Study the drawing (mm; zero at the part's minimum x, y, z) and answer. A direction names the side the tool comes from. Coordinates: 2 decimals unless noted, no trailing zeros. Write each loop counter-clockwise with the first axis right and the second up, starting at its lowest first coordinate (ties: lowest second). Pieces come first, ordered by that corner, then holes. Notation, with made-up numbers: (51, 69.5) -> (110, 69.5) arc R15 ccw to (110, 87.5) -> close; hole circle Ø5 at (-22, 66). An arc over 180 degrees is marked (long way). Write item = value, one per line. Start each with the question number.
1) Section C-C (x = 15) is taken. Determine the outline of the cut face in (y, z).
2) Flat-ended cylindrical pins translate along their axes: pin 1 Ø2 at (x, z) = (18.5, 16) entering from -Y; pin 2 Ø1.5 at (x, y) = (12, 19) entering from -Z; pin 3 Ø6.5 at (y, z) = (32, 10) entering from -X; pin 4 Ø4.5 at (x, z) = (17.5, 9.5) entering from -Y. Find the tip coordinate at first contact, or state that the pin passes through.
3) Section A-A (y = 43) is taken. Determine the outline of the cut face in (x, z).
4) Section B-B (z = 10) is taken. Determine the outline of the cut face in (x, y), plus the area to 3 significant figures.
5) Section D-D (x = 4.75) is taken. Determine the outline of the cut face in (y, z).
6) Find the intervals of material crossed by line 1 along Y through (x, z) = (9.5, 10); line 2 along Y through (x, z) = (11.25, 9); line 3 along Y through (x, z) = (22, 14.5), in increasing order. Write a range as from..to.
7) For a pull along X with two mould halves and no side action, classify the marked faces 3, 4 and 5 as released by +X, released by -X, zero draft, split by the parting line, or undercut.
8) A tool of negligible diameter and unlimited length cuts with its end or side. For the marked faces 1 and 2, from which of +Z, -Z, +X, -X, +Y, -Y can it reach the whole face along a straight path? Write none if from no direction.
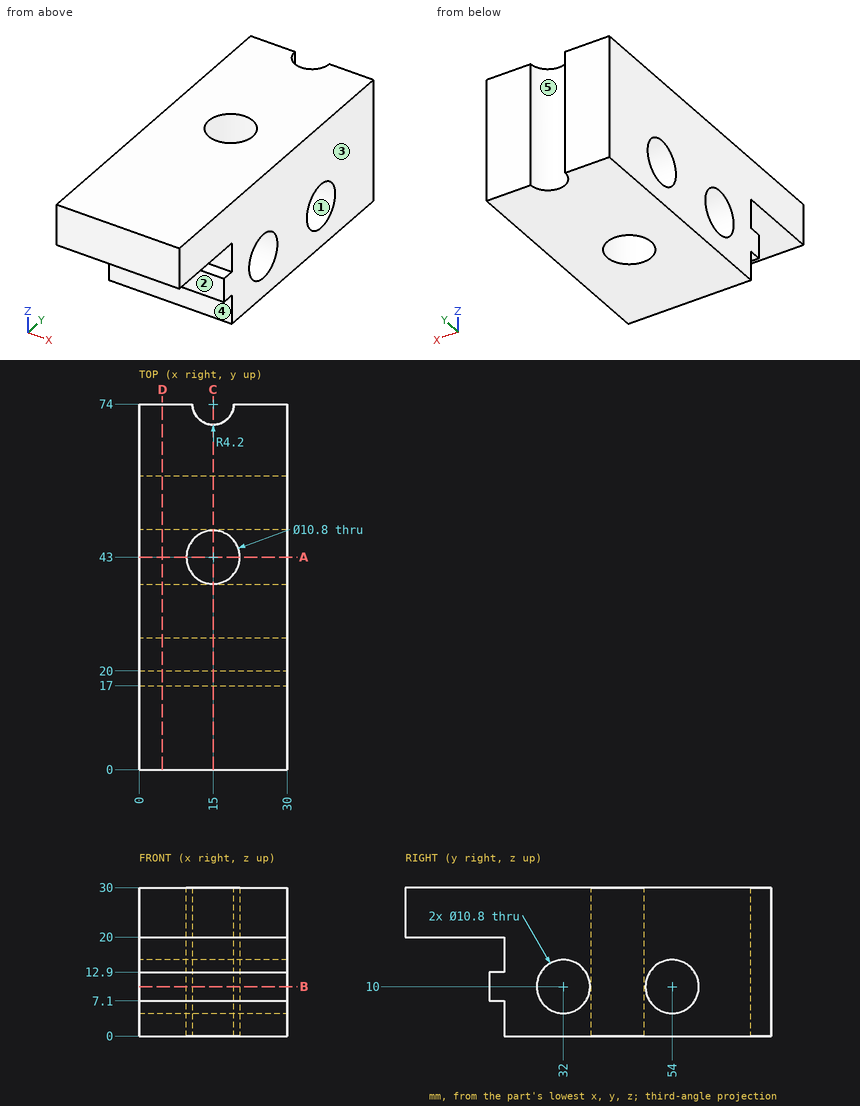
Answer key:
q1.outline = (0, 20) -> (20, 20) -> (20, 12.9) -> (17, 12.9) -> (17, 7.1) -> (20, 7.1) -> (20, 0) -> (37.6, 0) -> (37.6, 30) -> (0, 30) -> close; (48.4, 0) -> (69.8, 0) -> (69.8, 30) -> (48.4, 30) -> close; hole circle Ø10.8 at (32, 10); hole circle Ø10.8 at (54, 10)
q2.pin_1 = 20
q2.pin_2 = 7.1
q2.pin_3 = through
q2.pin_4 = 17
q3.outline = (0, 0) -> (9.6, 0) -> (9.6, 30) -> (0, 30) -> close; (20.4, 0) -> (30, 0) -> (30, 30) -> (20.4, 30) -> close
q4.outline = (0, 17) -> (30, 17) -> (30, 26.6) -> (0, 26.6) -> close; (0, 37.4) -> (30, 37.4) -> (30, 48.6) -> (0, 48.6) -> close; (0, 59.4) -> (30, 59.4) -> (30, 74) -> (19.2, 74) arc R4.2 cw to (10.8, 74) -> (0, 74) -> close; hole circle Ø10.8 at (15, 43)
q4.area = 943 mm^2
q5.outline = (0, 20) -> (20, 20) -> (20, 12.9) -> (17, 12.9) -> (17, 7.1) -> (20, 7.1) -> (20, 0) -> (74, 0) -> (74, 30) -> (0, 30) -> close; hole circle Ø10.8 at (32, 10); hole circle Ø10.8 at (54, 10)
q6.line_1 = 17..26.6, 37.4..48.6, 59.4..74
q6.line_2 = 17..26.69, 37.31..39.11, 46.89..48.69, 59.31..72.11
q6.line_3 = 20..29.02, 34.98..51.02, 56.98..74
q7.face_3 = released by +X
q7.face_4 = zero draft
q7.face_5 = undercut
q8.face_1 = +X, -X
q8.face_2 = -Z, +X, -X, -Y
